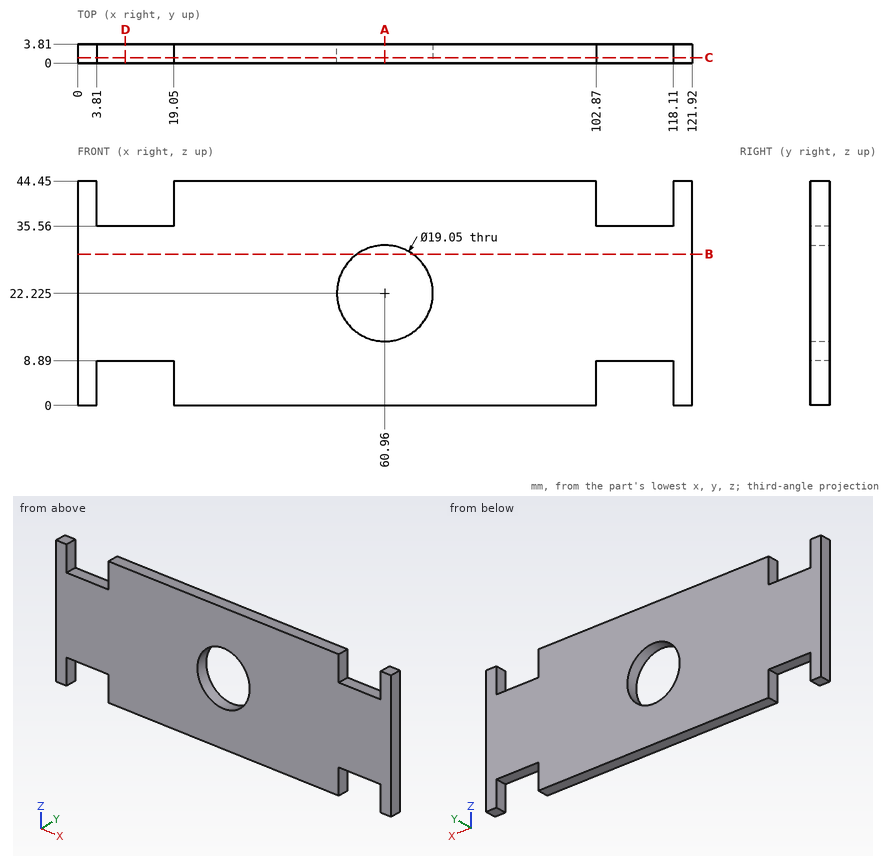
Design review of the part shown in the three views and the two pictorial views. Dimensions are in mm from the part's minimum x, y and z. Round coordinates to 2 decimals unless told otherwise and drop trailing zeros. Order: outer loops, then holes, each group sorted by start corner. A loop starts at its lowest first (then second) coordinate and runs counter-clockwise, first axis right, second up.
(1) Wall thickness on L1, parallel to X at y = 2.6, z = 38.5; L2, parallel to Z at x = 60.96, y = 2.25; L3, parallel to Z at x = 113.5, y = 1.75: over which ranges is each line inside the solid? List them lowest first.
Working result:
L1: x = 0 to 3.81, 19.05 to 102.87, 118.11 to 121.92
L2: z = 0 to 12.7, 31.75 to 44.45
L3: z = 8.89 to 35.56
(2) Take a section at D-D, the plane x = 9.5. State the section outline as (y, z) points.
Working result:
outline: (0, 8.89) - (3.81, 8.89) - (3.81, 35.56) - (0, 35.56) - close
(3) Take a section at A-A, the plane x = 60.96. State the section outline as (y, z) points.
Working result:
outline: (0, 0) - (3.81, 0) - (3.81, 12.7) - (0, 12.7) - close; (0, 31.75) - (3.81, 31.75) - (3.81, 44.45) - (0, 44.45) - close
(4) Take a section at B-B, the plane z = 30. State the section outline as (x, y) points.
Working result:
outline: (0, 0) - (55.46, 0) - (55.46, 3.81) - (0, 3.81) - close; (66.46, 0) - (121.92, 0) - (121.92, 3.81) - (66.46, 3.81) - close
(5) For P1, Ø1.9, axis at x = 9, y = 2.5, coming from the -Z side, flat-tipped, find the tip position at first contact; note if it passes through.
Working result:
P1: stops at z = 8.89
(6) Take a section at C-C, the plane y = 1.1. State the section outline as (x, z) points (3 decimals).
Working result:
outline: (0, 0) - (3.81, 0) - (3.81, 8.89) - (19.05, 8.89) - (19.05, 0) - (102.87, 0) - (102.87, 8.89) - (118.11, 8.89) - (118.11, 0) - (121.92, 0) - (121.92, 44.45) - (118.11, 44.45) - (118.11, 35.56) - (102.87, 35.56) - (102.87, 44.45) - (19.05, 44.45) - (19.05, 35.56) - (3.81, 35.56) - (3.81, 44.45) - (0, 44.45) - close; hole circle Ø19.05 at (60.96, 22.225)
